Check sheet for the drawn part. Datum: minimum x, y, z corner. Units: mm. A direction names the side the tool comes from. Coordinates: 2 decimals unless noted, no trailing zeros. Write each loop counter-clockwise with the first axis right and the second up, starting at its lowest first coordinate (ties: lowest second). Pieces come first, ordered by that corner, then holes. Notation, with made-up numbers: M -35.75,-2 L -16.75,-2 A23 ccw -16.75,34 Z; hole C 60,69.25 d11. An arc over 180 degrees is marked long. Answer as CSV lines item,"result". Start each with the question number.
Q1. Sectioned sample at D-D, the plane z = 7.75. Record the cut outline in (x, y), then the cut area to 3 significant figures.
Q2. Sectioned sample at B-B, the plane z = 3. Record the cut outline in (x, y), then the cut area to 3 significant figures.
Q3. Thickness scan on line 1 along X through (y, z) = (17.55, 6); line 2 along Y through (x, z) = (12, 3); line 3 along X through (y, z) = (6, 11). Record the ranges inside material, lowest first. Write a range as from..to.
Q4. Access from +Z, -Z, +X, -X, +Y, -Y to the whole of each face (thin tool, end or side, straight path). Record for the marked faces 1, 2, 3 and 4.
Q5. Sectioned sample at C-C, the plane y = 24.75. Record the cut outline in (x, z).
Q6. Sectioned sample at A-A, the plane x = 2.5. Record the cut outline in (y, z).
Q7. Depth check by flat-ended pin: pin 1 Ø1.5 at (x, z) = (29, 7) entering from +Y; pin 2 Ø1.2 at (y, z) = (21, 5) entering from +X; pin 3 Ø5 at (x, z) = (25, 9.5) entering from +Y; pin 4 Ø1.6 at (x, z) = (2.5, 6) entering from +Y (1 decimal). Enter the tip coordinate at first touch or a pass-through.
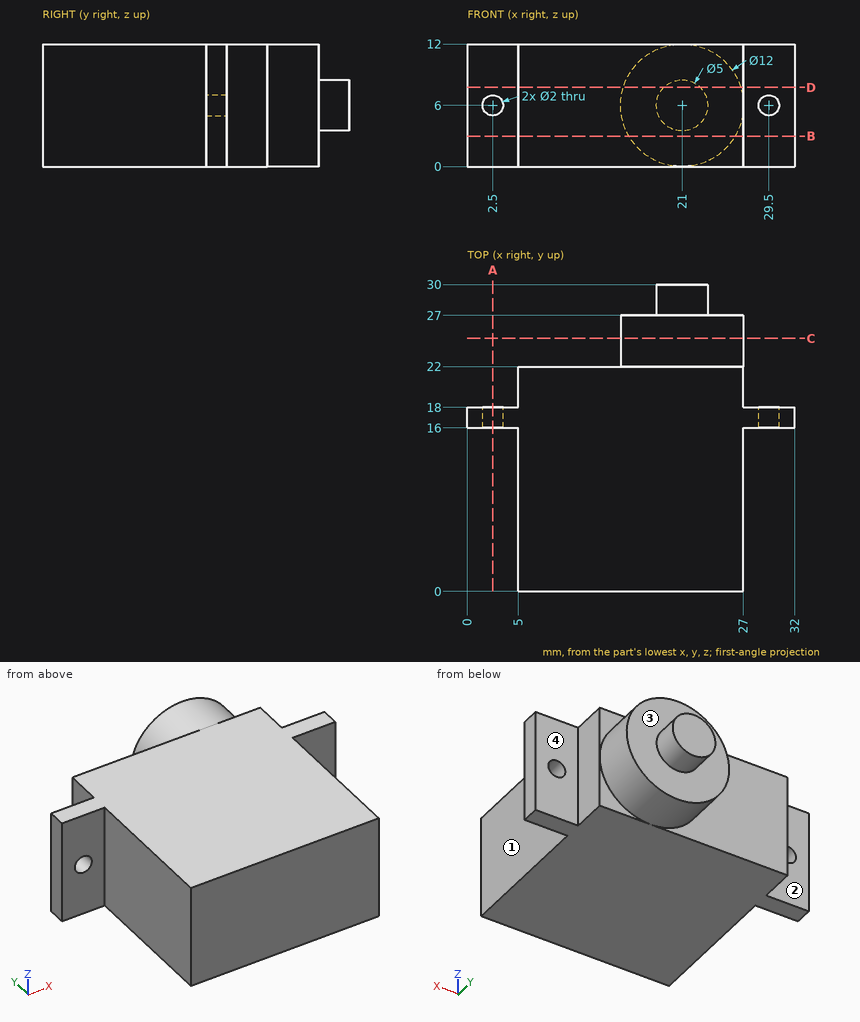
Output:
1,outline,"M 0,16 L 5,16 L 5,0 L 27,0 L 27,16 L 32,16 L 32,18 L 27,18 L 27,22 L 26.74,22 L 26.74,27 L 22.79,27 L 22.79,30 L 19.21,30 L 19.21,27 L 15.26,27 L 15.26,22 L 5,22 L 5,18 L 0,18 Z"
1,area,"572 mm^2"
2,outline,"M 0,16 L 5,16 L 5,0 L 27,0 L 27,16 L 32,16 L 32,18 L 27,18 L 27,22 L 26.2,22 L 26.2,27 L 15.8,27 L 15.8,22 L 5,22 L 5,18 L 0,18 Z"
2,area,"556 mm^2"
3,line 1,"x = 0..1.5, 3.5..28.5, 30.5..32"
3,line 2,"y = 0..22"
3,line 3,"x = 5..27"
4,face 1,"+Z, -Z, +X, -Y"
4,face 2,"+Z, -Z, -X, +Y"
4,face 3,"+Y"
4,face 4,"+Z, -Z, +X, +Y"
5,outline,"C 21,6 d12"
6,outline,"M 16,0 L 18,0 L 18,5 L 16,5 Z; M 16,7 L 18,7 L 18,12 L 16,12 Z"
7,pin 1,"stops at y = 18"
7,pin 2,"stops at x = 27"
7,pin 3,"stops at y = 27"
7,pin 4,"passes through"
